```python
from build123d import *

# Parameters (mm, degrees)
F0_W     = 101.6
F0_H     = 101.6
F1_DEPTH = 24.765
F2_W     = 19.05
F2_H     = 19.05
F3_DEPTH = 6.35
F2_R     = 12.7
F4_DEPTH = 12.7


with BuildPart() as f1:
    # F0 (on Top) → F1 (new body)
    with BuildSketch(Plane.XY):
        Rectangle(F0_W, F0_H)
    extrude(amount=F1_DEPTH)

    # F2 (on face) → F3 (cut)
    with BuildSketch(Plane.XY.offset(24.765)):
        with Locations((-28.575, 28.575)):
            Rectangle(F2_W, F2_H)
    extrude(amount=-F3_DEPTH, mode=Mode.SUBTRACT)

    # F2 (on face) → F4 (cut)
    with BuildSketch(Plane.XY.offset(24.765)):
        Circle(F2_R)
    extrude(amount=-F4_DEPTH, mode=Mode.SUBTRACT)


solid = f1.part
```
Part model, mm, in its own coordinate system. A direction names the side the tool comes from. Give positions to 0.01 mm unless a question says otherwise; leave off trailing zeros. Loops run counter-clockwise (first coordinate to the right, second up) from the corner with the lowest first, then second, coordinate; pieces in that order, holes last. Notation, with made-up numbers: M -15.5,42 L 31.5,42 A19 ccw 31.5,69 Z; hole C 55.25,35.5 d5. An arc over 180 degrees is marked long. Return JSON: item names as keys, results as strings.
1) Saw through at C-C, the plane z = 21.5. List the corners of the cut face in (x, y).
Calculated:
{"outline": "M -50.8,-50.8 L 50.8,-50.8 L 50.8,50.8 L -50.8,50.8 Z; hole M -38.1,19.05 L -19.05,19.05 L -19.05,38.1 L -38.1,38.1 Z; hole C 0,0 d25.4"}
2) Pull direction X, two halves, no side cores. Call faces 3 (the face through (11, -11, 24.765)), 4 (the face through (-38.1, 28, 22)), 5 (the face through (-50.8, -1, 12)): released by +X, released by -X, zero draft, split by the parting line, or undercut.
Calculated:
{"face 3": "zero draft", "face 4": "undercut", "face 5": "released by -X"}
3) Saw through at A-A, the plane y = 0. List the corners of the cut face in (x, z) (3 decimals).
Calculated:
{"outline": "M -50.8,0 L 50.8,0 L 50.8,24.765 L 12.7,24.765 L 12.7,12.065 L -12.7,12.065 L -12.7,24.765 L -50.8,24.765 Z"}
4) Flat gauge pins, fed straight in: pin 1 Ø10 at (x, y) = (-31.5, 15) entering from -Z; pin 2 Ø5.5 at (x, y) = (-30, 29) entering from +Z (3 decimals); pin 3 Ø7.5 at (x, y) = (1, 0) entering from +Z (3 decimals). Where does each tip first touch, or does it go through?
Calculated:
{"pin 1": "stops at z = 0", "pin 2": "stops at z = 18.415", "pin 3": "stops at z = 12.065"}
5) Drill centre lines: line 1 (Y direction, x = 0, z = 20.5); line 2 (Z direction, x = -38, y = 29) (3 decimals); line 3 (X direction, y = 4.5, z = 13.5). Where is each one in solid material? Low to high.
Calculated:
{"line 1": "y = -50.8 to -12.7, 12.7 to 50.8", "line 2": "z = 0 to 18.415", "line 3": "x = -50.8 to -11.88, 11.88 to 50.8"}
6) Saw through at D-D, the plane z = 15. List the corners of the cut face in (x, y), then the cut area to 3 significant figures.
Calculated:
{"outline": "M -50.8,-50.8 L 50.8,-50.8 L 50.8,50.8 L -50.8,50.8 Z; hole C 0,0 d25.4", "area": "9,820 mm2"}
7) 3-axis set-ups, long thin cutter, end or side, ignore diameter. For faces 1 (the face through (50.8, -1, 12)), 2 (the face through (-19.05, 28, 22)): which of +Z, -Z, +X, -X, +Y, -Y reach the whole face in a straight line?
Calculated:
{"face 1": "+Z, -Z, +X, +Y, -Y", "face 2": "+Z"}
